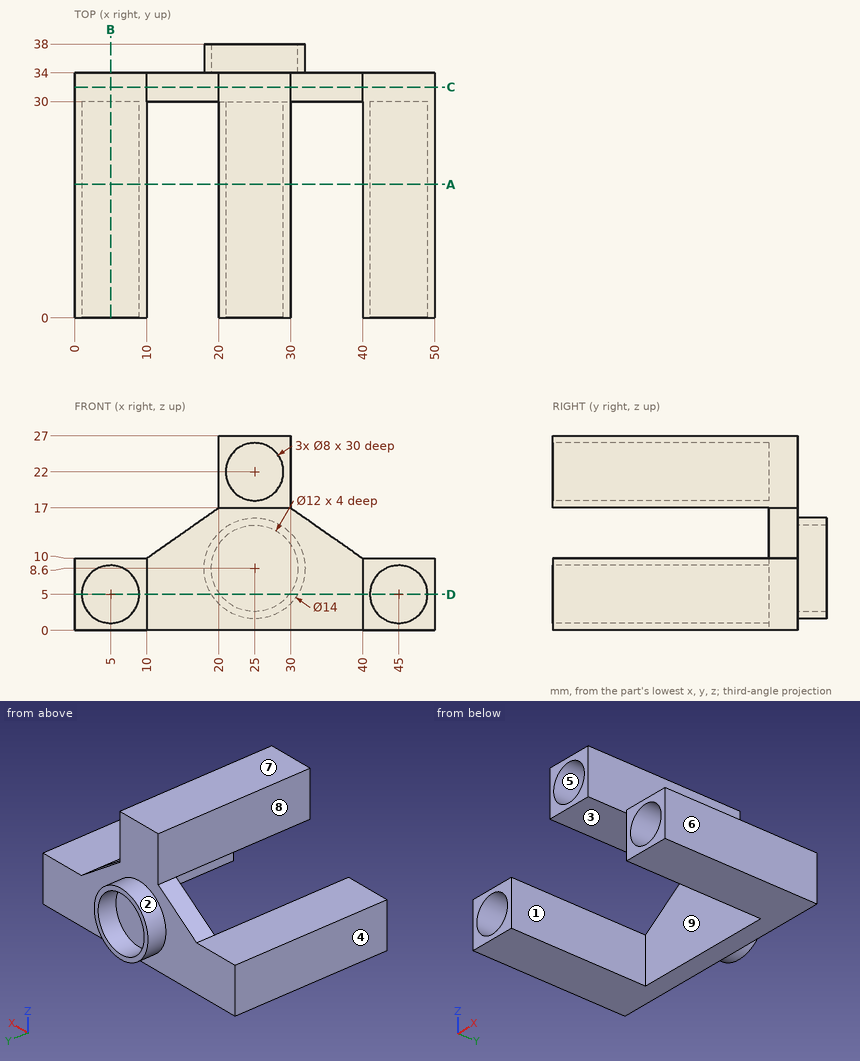
Answer from the drawing. Dimensions are ordinates in mm from the lowest x, y and z of the part. A direction names the side the tool comes from. Round coordinates to 2 decimals unless told otherwise and drop trailing zeros. Loops run counter-clockwise (first coordinate to the right, second up) from the corner with the lowest first, then second, coordinate; pieces in that order, holes last.
1) A cutting plane is placed at C-C on y = 32. Determine the outline of the cut face in (x, z).
Outcome:
outline: (0, 0) - (50, 0) - (50, 10) - (40, 10) - (30, 17) - (30, 27) - (20, 27) - (20, 17) - (10, 10) - (0, 10) - close
2) A cutting plane is placed at A-A on y = 18.5. Determine the outline of the cut face in (x, z).
Outcome:
outline: (0, 0) - (10, 0) - (10, 10) - (0, 10) - close; (20, 17) - (30, 17) - (30, 27) - (20, 27) - close; (40, 0) - (50, 0) - (50, 10) - (40, 10) - close; hole circle Ø8 at (5, 5); hole circle Ø8 at (25, 22); hole circle Ø8 at (45, 5)
3) A cutting plane is placed at D-D on z = 5. Determine the outline of the cut face in (x, y), plus the area to 3 significant figures.
Outcome:
outline: (0, 0) - (1, 0) - (1, 30) - (9, 30) - (9, 0) - (10, 0) - (10, 30) - (40, 30) - (40, 0) - (41, 0) - (41, 30) - (49, 30) - (49, 0) - (50, 0) - (50, 34) - (31, 34) - (31, 38) - (29.8, 38) - (29.8, 34) - (20.2, 34) - (20.2, 38) - (19, 38) - (19, 34) - (0, 34) - close
area: 330 mm2
4) For the marked faces 1, 2, 3, 4 and 5, determine the directions among +Z, -Z, +X, -X, +Y, -Y from which every point of the face is accessible in a straight line to the end or side of a thin tool.
Outcome:
face 1: +Z, -Z, -Y
face 2: +Y
face 3: -Z, +X, -X, -Y
face 4: +Z, -Z, -X, +Y, -Y
face 5: -Y
5) A cutting plane is placed at B-B on x = 5. Determine the outline of the cut face in (y, z), plus the area to 3 significant figures.
Outcome:
outline: (0, 0) - (34, 0) - (34, 10) - (0, 10) - (0, 9) - (30, 9) - (30, 1) - (0, 1) - close
area: 100 mm2
6) Given P1, Ø5, axis at x = 7.5, y = 16.5, coming from the +Z side; P2, Ø6.5, axis at x = 45, z = 5, coming from the -Y side; P3, Ø11, axis at x = 27, y = 20, coming from the -Z side; P4, Ø2, axis at x = 32.5, y = 13, coming from the -Z side, each flat-ended and moving along its own axis, determine where each tip first touches the part or whether it passes through.
Outcome:
P1: stops at z = 10
P2: stops at y = 30
P3: stops at z = 17
P4: passes through
7) Consider line 1 (Z direction, x = 25, y = 35); line 2 (X direction, y = 35.3, z = 8.6); line 3 (Z direction, x = 45, y = 11.5). Determine where each line is inside the solid, lowest interval first.
Outcome:
line 1: z = 1.6 to 2.6, 14.6 to 15.6
line 2: x = 18 to 19, 31 to 32
line 3: z = 0 to 1, 9 to 10
8) For a pull along X with two mould halves and no side action, classify the marked faces 6, 7, 8 and 9 as released by +X, released by -X, zero draft, split by the parting line, or undercut.
Outcome:
face 6: released by +X
face 7: zero draft
face 8: released by -X
face 9: undercut
